Part model, mm, in its own coordinate system. Face numbers are marked on the shaded views. A direction names the side the tool comes from. Coordinates: 2 decimals unless noted, no trailing zeros. Loops run counter-clockwise (first coordinate to the right, second up) from the corner with the lowest first, then second, coordinate; pieces in that order, holes last. Notation, with made-up numbers: M -30.5,16 L 24.5,16 A12 cw 24.5,22 Z; hole C 3.5,74.5 d2. An arc over 180 degrees is marked long. Use a Markdown table: item, result. Add a question column.
1) Tool access for the marked faces 1, 2 and 3: list every direction of +Z, -Z, +X, -X, +Y, -Y with a clear straight run to the whole face (end or side of a thin tool).
2) Band-saw the part on C-C (x = 128.5). List the corners of the cut face in (y, z), plus the area to 3 significant figures.
3) Pin check, flat tips, straight feed: pin 1 Ø12 at (x, y) = (168, 2) entering from +Z; pin 2 Ø12 at (x, z) = (132, -6) entering from -Y; pin 3 Ø8 at (x, z) = (142.5, 5.5) entering from -Y. Stop position of each tip, or through.
4) Wall check: probe 1 along X at (y, z) = (7.5, -7); probe 2 along Y at (x, z) = (20.5, 0); probe 3 along X at (y, z) = (-8.25, -3.75). Give the ranges that are in metal, low to high. Write a range as from..to.
5) Band-saw the part on D-D (x = 81). List the corners of the cut face in (y, z), plus the area to 3 significant figures.
from build123d import *

# Parameters (mm, degrees)
FILLET1_R     = 0.3
CHAMFER1_SIZE = 0.5


with BuildPart() as part:
    # Sketch1 → Revolve1 (revolve)
    with BuildSketch(Plane.XY, mode=Mode.PRIVATE) as revolve1_sk:
        Polygon((0, 0), (200, 0), (200, 7.5), (173, 7.5), (173, 10), (100, 10), (100, 12.5), (18, 12.5), (18, 10), (4, 10), (4, 9.5), (2.65, 9.5), (2.65, 10), (0, 10), align=None)
    revolve(revolve1_sk.sketch.rotate(Axis((0, 0, 0), (1, 0, 0)), 90), axis=Axis((0, 0, 0), (1, 0, 0)))

    # Fillet1
    fillet1_edges = [part.edges().sort_by_distance(p)[0] for p in [
        (100, 0, -10),
        (18, 0, -10),
    ]]
    fillet(fillet1_edges, radius=FILLET1_R)

    # Chamfer1
    chamfer1_edges = [part.edges().sort_by_distance(p)[0] for p in [
        (200, 0, -7.5),
        (0, 0, -10),
    ]]
    chamfer(chamfer1_edges, length=CHAMFER1_SIZE)


solid = part.part
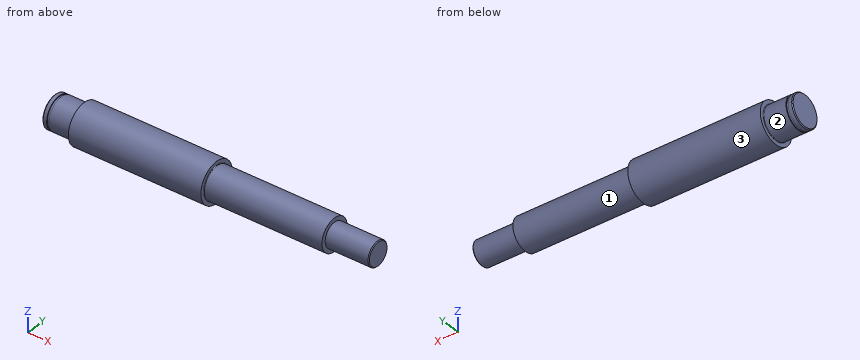
Entries:
| question | item | result |
|---|---|---|
| 1 | face 1 | +X |
| 1 | face 2 | -X |
| 1 | face 3 | +X, -X |
| 2 | outline | C 0,0 d20 |
| 2 | area | 314 mm2 |
| 3 | pin 1 | z = 10 |
| 3 | pin 2 | y = -10 |
| 3 | pin 3 | y = -9.89 |
| 4 | probe 1 | 18..100 |
| 4 | probe 2 | -12.5..12.5 |
| 4 | probe 3 | 0..173 |
| 5 | outline | C 0,0 d25 |
| 5 | area | 491 mm2 |
